Read the model definition and answer for the solid it produces. Units are mm, in the model's axes. A direction names the side the tool comes from. Give positions to 0.01 mm unless a question says otherwise; leave off trailing zeros. Write each loop counter-clockwise with the first axis right and the second up, starting at its lowest first coordinate (ties: lowest second). Pieces come first, ordered by that corner, then holes. Notation, with made-up numbers: M 56,77 L 109,77 A15 ccw 109,94 Z; hole C 83,-5.5 d6. An arc over 180 degrees is marked long. Use a Markdown table: item, result. Add a question column.
Item 1: For faces 4 (the flat face through (0, 18, 2)), 5 (the flat face through (-8, -22, 1.2)), 6 (the flat face through (-7.7, -21.6, 0.6)), 7 (the flat face through (-9.2, -23.4, 0.6)), 8 (the flat face through (-8.5, -23.4, 0.6)), determine the directions among +Z, -Z, +X, -X, +Y, -Y from which every point of the face is accessible in a straight line to the end or side of a thin tool.
Item 2: Consider probe 1 along Y at (x, z) = (-16, 0.35); probe 2 along Y at (x, z) = (-9, 3.1); probe 3 along Z at (x, y) = (15.5, -11.5). Determine where each line is inside the solid, lowest interval first. Write a range as [from, to].
Item 3: A cutting plane is placed at D-D on x = -8. Determine the outline of the cut face in (y, z).
Item 4: The mould has two halves that part along X. Classify faces 1 (the flat face through (0, -17, 2)), 2 (the flat face through (-7.7, -22.1, 0.6)), 3 (the flat face through (-17.3, 0, 2)): pulls with the +X half, pulls with the -X half, needs draft (parallel to the pull), parting line crosses it, or undercut.
Item 5: Given P1, Ø0.7, axis at x = -8.5, z = 0.5, coming from the -Y side; P2, Ø0.7, axis at x = -6, z = 1.5, coming from the +Y side; P3, Ø12, axis at x = -4.5, y = 0.5, coming from the -Z side; P4, Ø0.5, axis at x = -7, z = 3, coming from the -Y side, each flat-ended and moving along its own axis, determine where each tip first touches the part or whether it passes through.
Item 6: A cutting plane is placed at A-A on x = 5. Determine the outline of the cut face in (y, z).
Item 7: A cutting plane is placed at B-B on y = -12. Determine the outline of the cut face in (x, z), then the cut area to 3 significant figures.
Item 8: A cutting plane is placed at C-C on y = 7. Determine the outline of the cut face in (x, z).
from build123d import *

# Parameters (mm, degrees)
SKETCH1_W           = 36.4
SKETCH1_H           = 37
BOSS_EXTRUDE1_DEPTH = 1
SKETCH2_W           = 34.6
SKETCH2_H           = 27.5
BOSS_EXTRUDE2_DEPTH = 2.2
SKETCH3_W           = 34.6
SKETCH3_H           = 7.5
BOSS_EXTRUDE3_DEPTH = 1.2
BOSS_EXTRUDE4_DEPTH = 0.2
SKETCH5_W           = 3
SKETCH5_H           = 3.5
SKETCH5_W_2         = 1.6
SKETCH5_H_2         = 2.5
BOSS_EXTRUDE5_DEPTH = 0.9


with BuildPart() as part:
    # Sketch1 → Boss-Extrude1 (new body)
    with BuildSketch(Plane.XY):
        Rectangle(SKETCH1_W, SKETCH1_H)
    extrude(amount=BOSS_EXTRUDE1_DEPTH)

    # Sketch2 → Boss-Extrude2 (add)
    with BuildSketch(Plane.XY.offset(1)):
        with Locations((0, 4.25)):
            Rectangle(SKETCH2_W, SKETCH2_H)
    extrude(amount=BOSS_EXTRUDE2_DEPTH)

    # Sketch3 → Boss-Extrude3 (add)
    with BuildSketch(Plane.XY.offset(1)):
        with Locations((0, -13.25)):
            Rectangle(SKETCH3_W, SKETCH3_H)
    extrude(amount=BOSS_EXTRUDE3_DEPTH)

    # Sketch4 → Boss-Extrude4 (add)
    with BuildSketch(Plane.XY.offset(1)):
        Polygon((-10.2, -17), (-6.7, -17), (-6.7, -20.6), (-4.7, -20.6), (-4.7, -26.1), (-10.7, -26.1), (-10.7, -20.6), (-10.2, -20.6), align=None)
    extrude(amount=BOSS_EXTRUDE4_DEPTH)

    # Sketch5 → Boss-Extrude5 (add)
    with BuildSketch(Plane(origin=(0, 0, 1), x_dir=(-1, 0, 0), z_dir=(0, 0, -1))):
        with Locations((7.7, -23.35)):
            Rectangle(SKETCH5_W, SKETCH5_H)
        with Locations((7.7, -23.35)):
            Rectangle(SKETCH5_W_2, SKETCH5_H_2, mode=Mode.SUBTRACT)
    extrude(amount=BOSS_EXTRUDE5_DEPTH)


solid = part.part
Filled in:
| question | item | result |
|---|---|---|
| 1 | face 4 | +Z, +X, -X, +Y |
| 1 | face 5 | +Z, +X, -X, -Y |
| 1 | face 6 | -Z, +X, -X |
| 1 | face 7 | -Z, -X, -Y |
| 1 | face 8 | -Z |
| 2 | probe 1 | [-18.5, 18.5] |
| 2 | probe 2 | [-9.5, 18] |
| 2 | probe 3 | [0, 2.2] |
| 3 | outline | M -26.1,1 L -25.1,1 L -25.1,0.1 L -24.6,0.1 L -24.6,1 L -22.1,1 L -22.1,0.1 L -21.6,0.1 L -21.6,1 L -18.5,1 L -18.5,0 L 18.5,0 L 18.5,1 L 18,1 L 18,3.2 L -9.5,3.2 L -9.5,2.2 L -17,2.2 L -17,1.2 L -26.1,1.2 Z |
| 4 | face 1 | needs draft |
| 4 | face 2 | undercut |
| 4 | face 3 | pulls with the -X half |
| 5 | P1 | y = -25.1 |
| 5 | P2 | y = 18 |
| 5 | P3 | z = 0 |
| 5 | P4 | y = -9.5 |
| 6 | outline | M -18.5,0 L 18.5,0 L 18.5,1 L 18,1 L 18,3.2 L -9.5,3.2 L -9.5,2.2 L -17,2.2 L -17,1 L -18.5,1 Z |
| 7 | outline | M -18.2,0 L 18.2,0 L 18.2,1 L 17.3,1 L 17.3,2.2 L -17.3,2.2 L -17.3,1 L -18.2,1 Z |
| 7 | area | 77.9 mm² |
| 8 | outline | M -18.2,0 L 18.2,0 L 18.2,1 L 17.3,1 L 17.3,3.2 L -17.3,3.2 L -17.3,1 L -18.2,1 Z |
